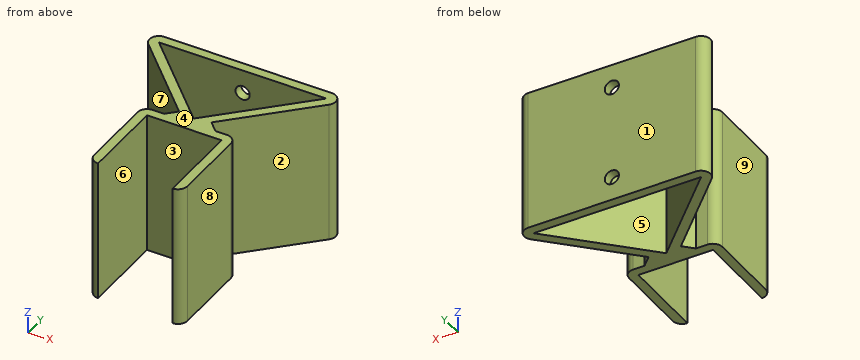
from build123d import *
from OCP.BRepFilletAPI import BRepFilletAPI_MakeChamfer

# Parameters (mm, degrees)
BOSS_EXTRUDE1_DEPTH = 38.1
CHAMFER1_SIZE       = 2.54
BOSS_EXTRUDE2_DEPTH = 38.1
CHAMFER2_SIZE       = 5.08
CHAMFER2_SIZE2      = 3.592102448
FILLET1_R           = 2.54
CUT_EXTRUDE1_REACH  = 70.978
SKETCH3_R           = 1.905


with BuildPart() as part:
    # Sketch1 → Boss-Extrude1 (new body)
    with BuildSketch(Plane.XY):
        Polygon((0, -3.592102448), (28.582742751, 24.990640303), (-28.582742751, 24.990640303), align=None)
        Polygon((0, 0), (22.450640303, 22.450640303), (-22.450640303, 22.450640303), align=None, mode=Mode.SUBTRACT)
    extrude(amount=BOSS_EXTRUDE1_DEPTH)

    # Chamfer1
    chamfer1_edges = [part.edges().sort_by_distance(p)[0] for p in [
        (0, -3.592102448, 19.05),
    ]]
    chamfer(chamfer1_edges, length=CHAMFER1_SIZE)

    # Sketch2 → Boss-Extrude2 (add)
    with BuildSketch(Plane.XY.offset(38.1)):
        Polygon((0, -1.796051224), (12.5, -1.796051224), (12.5, -26.796051224), (10, -26.796051224), (10, -24.296051224), (10, -4.296051224), (0, -4.296051224), (-10, -4.296051224), (-10, -24.296051224), (-10, -26.796051224), (-12.5, -26.796051224), (-12.5, -1.796051224), align=None)
    extrude(amount=-BOSS_EXTRUDE2_DEPTH)

    # Chamfer2: one chamfer whose edges measure the first distance from different faces: ONE call of the kernel's chamfer builder (chamfer() names one face for all edges)
    chamfer2_edges_1 = [part.edges().sort_by_distance(p)[0] for p in [
        (-1.796051224, -1.796051224, 19.05),
    ]]
    chamfer2_side_1 = [part.faces().sort_by_distance(p)[0] for p in [
        (-7.148025612, -1.796051224, 19.05),
    ]]
    chamfer2_edges_2 = [part.edges().sort_by_distance(p)[0] for p in [
        (1.796051224, -1.796051224, 19.05),
    ]]
    chamfer2_side_2 = [part.faces().sort_by_distance(p)[0] for p in [
        (7.148025612, -1.796051224, 19.05),
    ]]
    chamfer2 = BRepFilletAPI_MakeChamfer(part.part.solid().wrapped)
    for e in chamfer2_edges_1:
        chamfer2.Add(CHAMFER2_SIZE, CHAMFER2_SIZE2, e.wrapped, chamfer2_side_1[0].wrapped)  # the first distance lies on this face
    for e in chamfer2_edges_2:
        chamfer2.Add(CHAMFER2_SIZE, CHAMFER2_SIZE2, e.wrapped, chamfer2_side_2[0].wrapped)  # the first distance lies on this face
    add(Compound.cast(chamfer2.Shape()), mode=Mode.REPLACE)

    # Fillet1
    # the kernel refuses this fillet: 2.54 mm, written as the material it takes off along each edge
    with BuildSketch(Plane(origin=(-12.5, -26.796051224, 44.45), x_dir=(1, 0, 0), z_dir=(0, 0, -1)), Plane(origin=(12.5, -1.796051224, 44.45), x_dir=(-1, 0, 0), z_dir=(0, 0, -1)), Plane(origin=(12.5, -26.796051224, 44.45), x_dir=(0, 1, 0), z_dir=(0, 0, -1))) as fillet1_piece_1:
        with BuildLine():
            CenterArc((FILLET1_R, -FILLET1_R), FILLET1_R, 90, 90)
            Line((0, -FILLET1_R), (0, 0))
            Line((0, 0), (FILLET1_R, 0))
        make_face()
    extrude(amount=50.8, mode=Mode.SUBTRACT)
    with BuildSketch(Plane(origin=(-12.5, -1.796051224, 44.45), x_dir=(1, 0, 0), z_dir=(0, 0, -1))) as fillet1_piece_2:
        with BuildLine():
            CenterArc((FILLET1_R, FILLET1_R), FILLET1_R, 180, 90)
            Line((0, FILLET1_R), (0, 0))
            Line((0, 0), (FILLET1_R, 0))
        make_face()
    extrude(amount=50.8, mode=Mode.SUBTRACT)
    with BuildSketch(Plane(origin=(-28.582742751, 24.990640303, -15.330256121), x_dir=(1, 0, 0), z_dir=(0, 0, 1)), Plane(origin=(28.582742751, 24.990640303, -15.330256121), x_dir=(-0.7071067811865476, -0.7071067811865476, 0), z_dir=(0, 0, 1))) as fillet1_piece_3:
        with BuildLine():
            CenterArc((FILLET1_R * 2.41421356237, -FILLET1_R), FILLET1_R, 90, 135)
            Line((FILLET1_R * 1.70710678119, -FILLET1_R * 1.70710678119), (0, 0))
            Line((0, 0), (FILLET1_R * 2.41421356237, 0))
        make_face()
    extrude(amount=68.760512242, mode=Mode.SUBTRACT)

    # Sketch3 → Cut-Extrude1 (cut, up to next)
    with BuildSketch(Plane(origin=(0, 24.990640303, 0), x_dir=(1, 0, 0), z_dir=(0, 1, 0)), mode=Mode.PRIVATE) as cut_extrude1_sk1:
        with Locations(Location((0, -31.75, 0), (0, 0, 180))):
            Circle(SKETCH3_R)
    cut_extrude1_tool1 = extrude(cut_extrude1_sk1.sketch, amount=-CUT_EXTRUDE1_REACH, mode=Mode.PRIVATE) & part.part
    # Sketch3 → Cut-Extrude1 (cut, up to next)
    with BuildSketch(Plane(origin=(0, 24.990640303, 0), x_dir=(1, 0, 0), z_dir=(0, 1, 0)), mode=Mode.PRIVATE) as cut_extrude1_sk2:
        with Locations(Location((0, -6.35, 0), (0, 0, 180))):
            Circle(SKETCH3_R)
    cut_extrude1_tool2 = extrude(cut_extrude1_sk2.sketch, amount=-CUT_EXTRUDE1_REACH, mode=Mode.PRIVATE) & part.part
    add(cut_extrude1_tool1.solids().sort_by_distance((0, 24.99064, 31.75))[0], mode=Mode.SUBTRACT)
    add(cut_extrude1_tool2.solids().sort_by_distance((0, 24.99064, 6.35))[0], mode=Mode.SUBTRACT)


solid = part.part
CAD build for the part. Positions are in the model's coordinates, mm. Face numbers are marked on the shaded views. A direction names the side the tool comes from. Give positions to 0.01 mm unless a question says otherwise; leave off trailing zeros. Loops run counter-clockwise (first coordinate to the right, second up) from the corner with the lowest first, then second, coordinate; pieces in that order, holes last. Notation, with made-up numbers: M 4.25,56.25 L 8.25,56.25 A11 cw 8.25,60.25 Z; hole C -33,22.25 d3. An arc over 180 degrees is marked long. Answer in a Markdown table with one row per item. Add a question column.
Item 1: Probe probe 1 along Z at (x, y) = (0, 24) (3 decimals); probe 2 along X at (y, z) = (-10, 33); probe 3 along Y at (x, z) = (-6.5, 26). List the from-to ranges inside material, lowest first.
Item 2: Drop flat-ended pins along their axis: P1, Ø6, axis at y = -14, z = 27.5, coming from the -X side; P2, Ø1.5, axis at y = 4, z = 24, coming from the -X side; P3, Ø1.5, axis at y = -7, z = 8.5, coming from the +X side; P4, Ø3, axis at x = -10.5, y = -18, coming from the -Z side. Give the stop position or say it passes through.
Item 3: Band-saw the part on B-B on z = 14. Give the cut face in (x, y).
Item 4: Tool access for the marked faces 5, 6, 7, 8 and 9: list every direction of +Z, -Z, +X, -X, +Y, -Y with a clear straight run to the whole face (end or side of a thin tool).
Item 5: Mould opens along Y. For the marked faces 1, 2, 3 and 4 say: +Y half, -Y half, draft (parallel to the pull), parting line (faces both ways), or undercut.
Item 6: Band-saw the part on A-A on y = -17. Give the cut face in (x, z), then the cut area to 4 significant figures.
Item 7: Band-saw the part on D-D on z = 31.75. Give the cut face in (x, y) (3 decimals), then the cut area to 3 significant figures.
Item 8: Band-saw the part on C-C on x = -5.5. Give the cut face in (y, z).
Reply:
| question | item | result |
|---|---|---|
| 1 | probe 1 | z = 0 to 4.445, 8.255 to 29.845, 33.655 to 38.1 |
| 1 | probe 2 | x = -12.5 to -10, 10 to 12.5 |
| 1 | probe 3 | y = -4.3 to -1.42, 2.91 to 6.5, 22.45 to 24.99 |
| 2 | P1 | stops at x = -12.5 |
| 2 | P2 | stops at x = -8.34 |
| 2 | P3 | stops at x = 12.5 |
| 2 | P4 | stops at z = 0 |
| 3 | outline | M -24.25,20.65 L -4.34,0.74 L -6.88,-1.8 L -9.96,-1.8 A2.54 ccw -12.5,-4.34 L -12.5,-24.26 A2.54 ccw -10,-26.8 L -10,-4.3 L 10,-4.3 L 10,-26.8 A2.54 ccw 12.5,-24.26 L 12.5,-4.34 A2.54 ccw 9.96,-1.8 L 6.88,-1.8 L 4.34,0.74 L 24.25,20.65 A2.54 ccw 22.45,24.99 L -22.45,24.99 A2.54 ccw Z; hole M -22.45,22.45 L 0,0 L 22.45,22.45 Z |
| 4 | face 5 | +Z, -Z |
| 4 | face 6 | +Z, -Z, -Y |
| 4 | face 7 | +Z, -Z, -X |
| 4 | face 8 | +Z, -Z, +X, -Y |
| 4 | face 9 | +Z, -Z, -X, -Y |
| 5 | face 1 | +Y half |
| 5 | face 2 | undercut |
| 5 | face 3 | -Y half |
| 5 | face 4 | draft |
| 6 | outline | M -12.5,0 L -10,0 L -10,38.1 L -12.5,38.1 Z; M 10,0 L 12.5,0 L 12.5,38.1 L 10,38.1 Z |
| 6 | area | 190.5 mm^2 |
| 7 | outline | M -24.247,20.655 L -4.336,0.744 L -6.876,-1.796 L -9.96,-1.796 A2.54 ccw -12.5,-4.336 L -12.5,-24.256 A2.54 ccw -10,-26.796 L -10,-4.296 L 10,-4.296 L 10,-26.796 A2.54 ccw 12.5,-24.256 L 12.5,-4.336 A2.54 ccw 9.96,-1.796 L 6.876,-1.796 L 4.336,0.744 L 24.247,20.655 A2.54 ccw 22.451,24.991 L 1.905,24.991 L 1.905,22.451 L 22.451,22.451 L 0,0 L -22.451,22.451 L -1.905,22.451 L -1.905,24.991 L -22.451,24.991 A2.54 ccw Z |
| 7 | area | 466 mm^2 |
| 8 | outline | M -4.3,0 L -0.42,0 L -0.42,38.1 L -4.3,38.1 Z; M 1.91,0 L 5.5,0 L 5.5,38.1 L 1.91,38.1 Z; M 22.45,0 L 24.99,0 L 24.99,38.1 L 22.45,38.1 Z |
